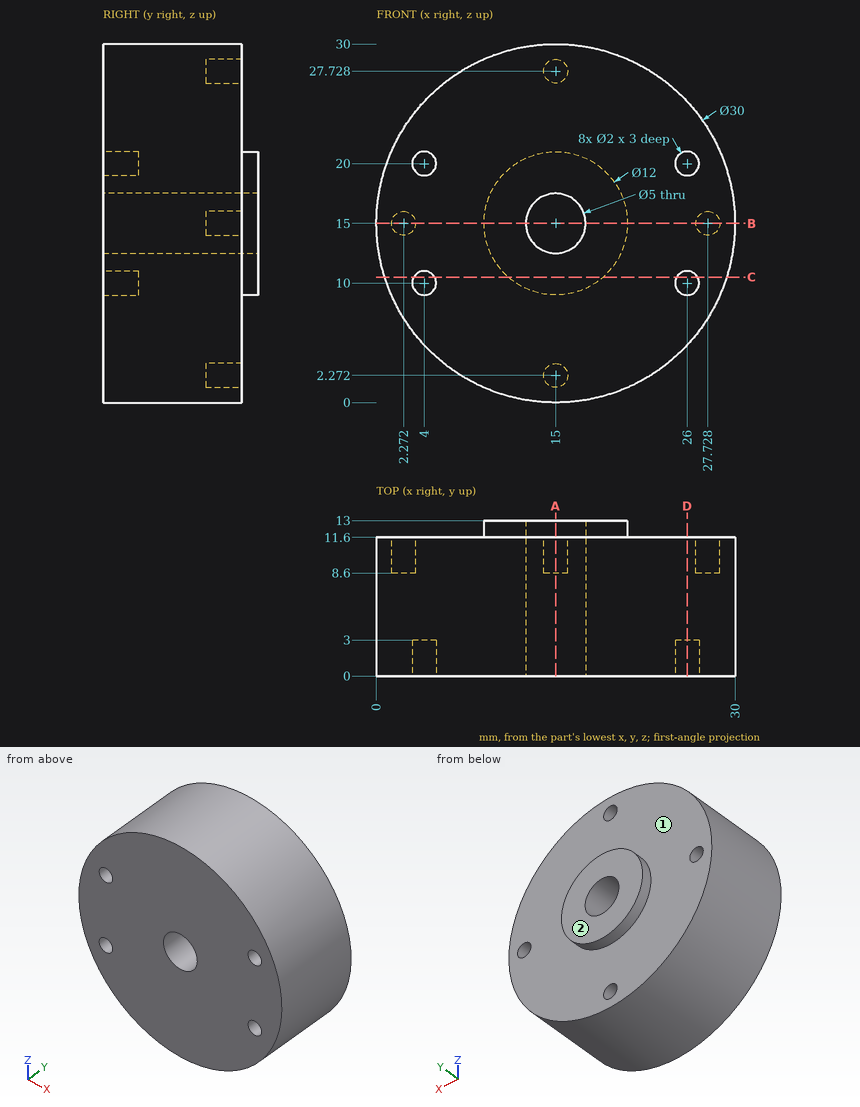
For this review, use the dimensioned drawing (mm, ordinates from the lowest corner) and the shaded views. A direction names the side the tool comes from. Give positions to 0.01 mm unless a question says otherwise; leave off trailing zeros. Order: outer loops, then holes, each group sorted by start corner. A loop starts at its lowest first (then second) coordinate and runs counter-clockwise, first axis right, second up. Notation, with made-up numbers: (79.5, 45.25) -> (99.5, 45.25) arc R18 ccw to (99.5, 50.25) -> close; hole circle Ø5 at (15, -12). An arc over 180 degrees is marked (long way). Write item = value, one per line. Start each with the question number.
(1) For L1, parallel to X at y = 2.35, z = 10; L2, parallel to X at y = 7.5, z = 15; L3, parallel to X at y = 2.5, z = 19.75, list the stretches that pass through material, from the lowest coordinate up. Write a range as from..to.
(2) For pin 1 Ø3 at (x, z) = (14.5, 6) entering from +Y; pin 2 Ø0.6 at (x, z) = (15, 2) entering from +Y; pin 3 Ø1 at (y, z) = (4.5, 3) entering from +X, all flat-tipped, find the tip position at first contact; note any pin that passes through.
(3) Take a section at A-A (x = 15). Write out the cut boundary in (y, z).
(4) Take a section at B-B (z = 15). Write out the cut boundary in (x, y).
(5) Tool access review of the marked faces 1 and 2: name each direction out of +Z, -Z, +X, -X, +Y, -Y from which nothing blocks a thin tool from reaching the whole face with its end or side.
(6) Take a section at C-C (z = 10.5). Write out the cut boundary in (x, y), plus the area to 3 significant figures.
(7) Take a section at D-D (x = 26). Write out the cut boundary in (y, z).
Returned:
q1.L1 = 0.86..3, 5..25, 27..29.14
q1.L2 = 0..12.5, 17.5..30
q1.L3 = 0.77..3.03, 4.97..25.03, 26.97..29.23
q2.pin_1 = 11.6
q2.pin_2 = 8.6
q2.pin_3 = 24.63
q3.outline = (0, 0) -> (11.6, 0) -> (11.6, 1.27) -> (8.6, 1.27) -> (8.6, 3.27) -> (11.6, 3.27) -> (11.6, 9) -> (13, 9) -> (13, 12.5) -> (0, 12.5) -> close; (0, 17.5) -> (13, 17.5) -> (13, 21) -> (11.6, 21) -> (11.6, 26.73) -> (8.6, 26.73) -> (8.6, 28.73) -> (11.6, 28.73) -> (11.6, 30) -> (0, 30) -> close
q4.outline = (0, 0) -> (12.5, 0) -> (12.5, 13) -> (9, 13) -> (9, 11.6) -> (3.27, 11.6) -> (3.27, 8.6) -> (1.27, 8.6) -> (1.27, 11.6) -> (0, 11.6) -> close; (17.5, 0) -> (30, 0) -> (30, 11.6) -> (28.73, 11.6) -> (28.73, 8.6) -> (26.73, 8.6) -> (26.73, 11.6) -> (21, 11.6) -> (21, 13) -> (17.5, 13) -> close
q5.face_1 = +Y
q5.face_2 = +Z, -Z, +X, -X, +Y
q6.outline = (0.69, 0) -> (3.13, 0) -> (3.13, 3) -> (4.87, 3) -> (4.87, 0) -> (25.13, 0) -> (25.13, 3) -> (26.87, 3) -> (26.87, 0) -> (29.31, 0) -> (29.31, 11.6) -> (18.97, 11.6) -> (18.97, 13) -> (11.03, 13) -> (11.03, 11.6) -> (0.69, 11.6) -> close
q6.area = 333 mm²
q7.outline = (0, 4.8) -> (11.6, 4.8) -> (11.6, 25.2) -> (0, 25.2) -> (0, 21) -> (3, 21) -> (3, 19) -> (0, 19) -> (0, 11) -> (3, 11) -> (3, 9) -> (0, 9) -> close
